Verification items for the finished model (mm, model axes). Give positions to 0.01 mm unless a question says otherwise; leave off trailing zeros. Write each loop counter-clockwise with the first axis right and the second up, starting at its lowest first coordinate (ties: lowest second). Pieces come first, ordered by that corner, then holes. Notation, with made-up numbers: M 26,-12.75 L 38,-12.75 A13 cw 38,7.25 Z; hole C 22.25,35 d3. An arc over 180 degrees is marked long. Write item = value, one per line.
from build123d import *

# Parameters (mm, degrees)
SKETCH_1_R          = 38.625
EXTRUDE_1_DEPTH     = 100
SKETCH_2_R          = 35
CUT_EXTRUDE_3_DEPTH = 5
FILLET_8_R          = 10
SKETCH_4_R          = 26.339745962
CUT_EXTRUDE_4_DEPTH = 97.665379301


with BuildPart() as part:
    # 草圖1 → 填料-伸長1 (new body)
    with BuildSketch(Plane(origin=(0, 0, 0), x_dir=(1, 0, 0), z_dir=(0, 1, 0))):
        with Locations(Location((0, 0, 0), (0, 0, 270))):
            Circle(SKETCH_1_R)
    extrude(amount=EXTRUDE_1_DEPTH)

    # 草圖2 → 除料-伸長3 (cut)
    with BuildSketch(Plane(origin=(0, 100, 0), x_dir=(1, 0, 0), z_dir=(0, 1, 0))):
        with Locations(Location((0, 0, 0), (0, 0, 270))):
            Circle(SKETCH_2_R)
    extrude(amount=-CUT_EXTRUDE_3_DEPTH, mode=Mode.SUBTRACT)

    # 圓角8
    # the kernel refuses this fillet: 10 mm, written as the material it adds along each edge
    with BuildSketch(Plane(origin=(0, 95, 0), x_dir=(0, 0, 1), z_dir=(-1, 0, 0))) as fillet_8_piece_1:
        with BuildLine():
            CenterArc((26.339745962, 10), FILLET_8_R, 270, 60)
            Line((26.339745962, 0), (26.339745962, -0.2))
            Line((26.339745962, -0.2), (35, -0.2))
            Line((35, -0.2), (35.2, 0))
            ThreePointArc((35.2, 0), (35.2, 2.5), (35.173205081, 4.9))
            Line((35.173205081, 4.9), (35, 5))
        make_face()
    revolve(axis=Axis((0, 95, 0), (0, 1, 0)))

    # 草圖4 → 除料-伸長4 (cut)
    with BuildSketch(Plane(origin=(0, 95, 0), x_dir=(1, 0, 0), z_dir=(0, 1, 0))):
        with Locations(Location((0, 0, 0), (0, 0, 270))):
            Circle(SKETCH_4_R)
    extrude(amount=-CUT_EXTRUDE_4_DEPTH, mode=Mode.SUBTRACT)


solid = part.part
1) Cross-section at B-B on z = 0. Record the boundary of the cut face in (x, y) (3 decimals), plus the area to 3 significant figures.
From the geometry:
outline = M -38.625,0 L -26.34,0 L -26.34,95 A10 cw -35,100 L -38.625,100 Z; M 26.34,0 L 38.625,0 L 38.625,100 L 35,100 A10 cw 26.34,95 Z
area = 2,400 mm^2
2) Material ranges on probe 1 along X at (y, z) = (20.5, 0) (3 decimals); probe 2 along Z at (x, y) = (0.5, 89.5) (3 decimals); probe 3 along Z at (x, y) = (-14.5, 22.5), recorded low to high. Write a range as from..to.
From the geometry:
probe_1 = -38.625..-26.34, 26.34..38.625
probe_2 = -38.622..-26.335, 26.335..38.622
probe_3 = -35.8..-21.99, 21.99..35.8
3) Depth check by flat-ended pin: P1, Ø10, axis at x = 14.5, z = 20.5, coming from the +Y side; P2, Ø3, axis at x = 15.5, y = 30, coming from the -Z side; P3, Ø1.5, axis at x = -25, y = 58.5, coming from the +Z side. Enter the tip coordinate at first touch or a pass-through.
From the geometry:
P1 = 95.74
P2 = -36
P3 = 30.06
4) Draft check along X on faces 1 (the flat face through (-25, 0, -9)), 2 (the cylindrical face through (-34.27, 49.3, 17.82)), 3 (the cylindrical face through (-25.713, 48.165, -5.71)). Enter one of: +X half, -X half, draft (parallel to the pull), parting line (faces both ways), or undercut.
From the geometry:
face_1 = draft
face_2 = parting line
face_3 = undercut
5) Cross-section at A-A on x = 0. Record the boundary of the cut face in (y, z) (3 decimals), plus the area to 3 significant figures.
From the geometry:
outline = M 0,-38.625 L 100,-38.625 L 100,-35 A10 cw 95,-26.34 L 0,-26.34 Z; M 0,26.34 L 95,26.34 A10 cw 100,35 L 100,38.625 L 0,38.625 Z
area = 2,400 mm^2
